Geometry: final body of the model. Coordinates: model frame, mm. A direction names the side the tool comes from. Give positions to 0.01 mm unless a question says otherwise; leave off trailing zeros. Write each loop counter-clockwise with the first axis right and the second up, starting at its lowest first coordinate (ties: lowest second). Pieces come first, ordered by that corner, then holes.
Q1. Line query: L1, parallel to Y at x = -35, z = 38.25; L2, parallel to Z at x = -33, y = 3.5; L3, parallel to Z at x = 1.55, y = 7.5. Output: solid intervals per line, ascending.
Q2. Cut plane C-C on y = 12.5. Return the cut outline in (x, z).
Q3. Pin query (flat end, axial travel): pin 1 (6 mm diameter, centred on y = 16.5, z = 34.5, fed in from -X); pin 2 (3.5 mm diameter, centred on y = 16, z = 29, fed in from +X); pin 3 (8.5 mm diameter, centred on x = -7.5, z = 12, fed in from +Y); pin 4 (0.9 mm diameter, centred on x = 19.5, z = 30, fed in from +Y). Return the tip coordinate at first contact, or that it passes through.
Q4. Cut plane A-A on y = 6. Return the cut outline in (x, z).
Q5. Cut plane D-D on z = 14.5. Return the cut outline in (x, y).
Q6. Draft query along Z for faces 1 (the face through (-23, 8, 37)), 2 (the face through (-11, 21, 17)), 3 (the face through (-36, 15, 39)). Return one class per face: pulls with the +Z half, pulls with the -Z half, needs draft (parallel to the pull), parting line crosses it, or undercut.
Q7. Cut plane B-B on x = -35. Return the cut outline in (y, z), plus the area to 3 significant figures.
Q8. Reachability of faces 4 (the face through (-0.5, 28, 19)), 5 (the face through (20, 8, 10)), 6 (the face through (-12, 18, 8)), 7 (the face through (0, 11, 20)), 8 (the face through (-11, 21, 20)) from +Z, -Z, +X, -X, +Y, -Y: full face, straight path, thin tool, end or side. Return the list, or none.
```python
from build123d import *

# Parameters (mm, degrees)
BOSS_EXTRUDE1_DEPTH     = 40
SKETCH2_R               = 1.5
BOSS_EXTRUDE2_DEPTH     = 5
SKETCH3_R               = 2.5
CUT_EXTRUDE1_DEPTH      = 50.497474683
CUT_EXTRUDE1_DEPTH_BACK = 50.497474683
SKETCH4_W               = 45
SKETCH4_H               = 15
BOSS_EXTRUDE3_DEPTH     = 3
SKETCH5_W               = 45
SKETCH5_H               = 15
BOSS_EXTRUDE4_DEPTH     = 3
SKETCH6_R               = 1.5
CUT_EXTRUDE2_DEPTH      = 63.04836823
CUT_EXTRUDE2_DEPTH_BACK = 63.04836823
SKETCH8_W               = 30
SKETCH8_H               = 40
SKETCH8_W_2             = 25
SKETCH8_H_2             = 10
BOSS_EXTRUDE7_DEPTH     = 3
BOSS_EXTRUDE8_DEPTH     = 3


with BuildPart() as part:
    # Sketch1 → Boss-Extrude1 (new body)
    with BuildSketch(Plane.XY):
        Polygon((0, 0), (25, 0), (25, 3), (3, 3), (3, 15), (0, 15), align=None)
    extrude(amount=BOSS_EXTRUDE1_DEPTH)

    # Sketch2 → Boss-Extrude2 (add)
    with BuildSketch(Plane(origin=(0, 3, 0), x_dir=(1, 0, 0), z_dir=(0, 1, 0))):
        with Locations((20, -10)):
            Circle(SKETCH2_R)
        with Locations((20, -30)):
            Circle(SKETCH2_R)
    extrude(amount=BOSS_EXTRUDE2_DEPTH)

    # Sketch3 → Cut-Extrude1 (cut, two sides)
    with BuildSketch(Plane.ZY) as cut_extrude1_sk:
        with Locations(Location((20, 7.5, 0), (0, 0, 270))):
            Circle(SKETCH3_R)
    extrude(amount=CUT_EXTRUDE1_DEPTH, mode=Mode.SUBTRACT)
    extrude(cut_extrude1_sk.sketch, amount=-CUT_EXTRUDE1_DEPTH_BACK, mode=Mode.SUBTRACT)

    # Sketch4 → Boss-Extrude3 (add)
    with BuildSketch(Plane(origin=(0, 0, 0), x_dir=(-1, 0, 0), z_dir=(0, 0, -1))):
        with Locations((22.5, 7.5)):
            Rectangle(SKETCH4_W, SKETCH4_H)
    extrude(amount=-BOSS_EXTRUDE3_DEPTH)

    # Sketch5 → Boss-Extrude4 (add)
    with BuildSketch(Plane.XY.offset(40)):
        with Locations((-22.5, 7.5)):
            Rectangle(SKETCH5_W, SKETCH5_H)
    extrude(amount=-BOSS_EXTRUDE4_DEPTH)

    # Sketch6 → Cut-Extrude2 (cut, two sides)
    with BuildSketch(Plane.XY.offset(40)) as cut_extrude2_sk:
        with Locations((-35, 12.5)):
            Circle(SKETCH6_R)
        with Locations((-35, 2.5)):
            Circle(SKETCH6_R)
    extrude(amount=CUT_EXTRUDE2_DEPTH, mode=Mode.SUBTRACT)
    extrude(cut_extrude2_sk.sketch, amount=-CUT_EXTRUDE2_DEPTH_BACK, mode=Mode.SUBTRACT)

    # Sketch8 → Boss-Extrude7 (add)
    with BuildSketch(Plane(origin=(0, 15, 0), x_dir=(1, 0, 0), z_dir=(0, 1, 0))):
        with Locations((-12, -20)):
            Rectangle(SKETCH8_W, SKETCH8_H)
        with Locations((-12, -30)):
            Rectangle(SKETCH8_W_2, SKETCH8_H_2, mode=Mode.SUBTRACT)
    extrude(amount=BOSS_EXTRUDE7_DEPTH)

    # 3DSketch1 → Boss-Extrude8 (add)
    with BuildSketch(Plane(origin=(-27, 18, 20), x_dir=(0.8320502943378437, 0.5547001962252291, 0), z_dir=(0, 0, -1))):
        Polygon((0, 0), (24.96150883, 16.641005887), (36.055512755, 0), (11.094003925, -16.641005887), align=None)
        Polygon((11.78737917, -11.371354023), (30.92453594, 1.386750491), (24.268133585, 11.371354023), (5.130976815, -1.386750491), align=None, mode=Mode.SUBTRACT)
    extrude(amount=BOSS_EXTRUDE8_DEPTH)


solid = part.part
```
Data:
1. L1: y = 0 to 1, 4 to 11, 14 to 15
1. L2: z = 0 to 3, 37 to 40
1. L3: z = 0 to 17.5, 22.5 to 40
2. outline: (-45, 0) - (-36.5, 0) - (-36.5, 3) - (-45, 3) - close; (-45, 37) - (-36.5, 37) - (-36.5, 40) - (-45, 40) - close; (-33.5, 0) - (3, 0) - (3, 40) - (-33.5, 40) - (-33.5, 37) - (0, 37) - (0, 3) - (-33.5, 3) - close
3. pin 1: stops at x = -45
3. pin 2: stops at x = 3
3. pin 3: stops at y = 18
3. pin 4: stops at y = 8
4. outline: (-45, 0) - (3, 0) - (3, 18) - (0, 18) - (0, 3) - (-45, 3) - close; (-45, 37) - (0, 37) - (0, 22) - (3, 22) - (3, 40) - (-45, 40) - close; circle Ø3 at (20, 10); circle Ø3 at (20, 30)
5. outline: (-27, 15) - (0, 15) - (0, 0) - (25, 0) - (25, 3) - (3, 3) - (3, 18) - (-27, 18) - close
6. face 1: undercut
6. face 2: pulls with the -Z half
6. face 3: needs draft
7. outline: (0, 0) - (1, 0) - (1, 3) - (0, 3) - close; (0, 37) - (1, 37) - (1, 40) - (0, 40) - close; (4, 0) - (11, 0) - (11, 3) - (4, 3) - close; (4, 37) - (11, 37) - (11, 40) - (4, 40) - close; (14, 0) - (15, 0) - (15, 3) - (14, 3) - close; (14, 37) - (15, 37) - (15, 40) - (14, 40) - close
7. area: 54.0 mm2
8. face 4: +Z, -Z
8. face 5: +Z, -Z, +X, +Y
8. face 6: -Z, +X, -X, +Y
8. face 7: -X, -Y
8. face 8: +Z, +X, -X, +Y
